```python
from build123d import *

# Parameters (mm, degrees)
SKETCH1_R             = 35
BOSS_EXTRUDE1_DEPTH   = 10
CUT_EXTRUDE1_REACH    = 52.498
SKETCH2_R             = 2.05
F_8_0MM_DOWEL_HOLE1_D = 8
M6_CLEARANCE_HOLE1_D  = 6.4


with BuildPart() as part:
    # Sketch1 → Boss-Extrude1 (new body)
    with BuildSketch(Plane(origin=(0, 0, 0), x_dir=(1, 0, 0), z_dir=(0, 1, 0))):
        with Locations(Location((0, 0, 0), (0, 0, 270))):
            Circle(SKETCH1_R)
    extrude(amount=-BOSS_EXTRUDE1_DEPTH)

    # Sketch2 → Cut-Extrude1 (cut, up to next)
    with BuildSketch(Plane(origin=(0, 0, 0), x_dir=(1, 0, 0), z_dir=(0, 1, 0)), mode=Mode.PRIVATE) as cut_extrude1_sk1:
        with Locations(Location((8.660254038, -5, 0), (0, 0, 270))):
            Circle(SKETCH2_R)
    cut_extrude1_tool1 = extrude(cut_extrude1_sk1.sketch, amount=-CUT_EXTRUDE1_REACH, mode=Mode.PRIVATE) & part.part
    # Sketch2 → Cut-Extrude1 (cut, up to next)
    with BuildSketch(Plane(origin=(0, 0, 0), x_dir=(1, 0, 0), z_dir=(0, 1, 0)), mode=Mode.PRIVATE) as cut_extrude1_sk2:
        with Locations(Location((0, 10, 0), (0, 0, 270))):
            Circle(SKETCH2_R)
    cut_extrude1_tool2 = extrude(cut_extrude1_sk2.sketch, amount=-CUT_EXTRUDE1_REACH, mode=Mode.PRIVATE) & part.part
    # Sketch2 → Cut-Extrude1 (cut, up to next)
    with BuildSketch(Plane(origin=(0, 0, 0), x_dir=(1, 0, 0), z_dir=(0, 1, 0)), mode=Mode.PRIVATE) as cut_extrude1_sk3:
        with Locations(Location((-8.660254038, -5, 0), (0, 0, 270))):
            Circle(SKETCH2_R)
    cut_extrude1_tool3 = extrude(cut_extrude1_sk3.sketch, amount=-CUT_EXTRUDE1_REACH, mode=Mode.PRIVATE) & part.part
    add(cut_extrude1_tool1.solids().sort_by_distance((8.660254, 0, 5))[0], mode=Mode.SUBTRACT)
    add(cut_extrude1_tool2.solids().sort_by_distance((0, 0, -10))[0], mode=Mode.SUBTRACT)
    add(cut_extrude1_tool3.solids().sort_by_distance((-8.660254, 0, 5))[0], mode=Mode.SUBTRACT)

    # Ø8.0mm Dowel Hole1 (through all)
    with Locations(Plane(origin=(0, -10, 0), x_dir=(-1, 0, 0), z_dir=(0, -1, 0))):
        with Locations((-13.75, 23.815698604), (13.75, -23.815698604)):
            Hole(F_8_0MM_DOWEL_HOLE1_D / 2)

    # M6 Clearance Hole1 (through all)
    with Locations(Plane(origin=(0, -10, 0), x_dir=(-1, 0, 0), z_dir=(0, -1, 0))):
        with Locations((-21.650635095, -12.5), (21.650635095, -12.5), (0, 25)):
            Hole(M6_CLEARANCE_HOLE1_D / 2)


solid = part.part
```
Could you check a few things on this model? Use its own coordinates, in mm. Round coordinates to 2 decimals unless told otherwise and drop trailing zeros. Write each loop counter-clockwise with the first axis right and the second up, starting at its lowest first coordinate (ties: lowest second). Pieces come first, ordered by that corner, then holes.
(1) If I drill on probe 1 along X at (y, z) = (-6.75, -24); probe 2 along X at (y, z) = (-4.75, -26); probe 3 along Z at (x, y) = (-21.5, -3.25), over which ranges is the centre line in solid material (lowest first)?
Findings below:
probe 1: x = -25.48 to -3.04, 3.04 to 9.75, 17.75 to 25.48
probe 2: x = -23.43 to -3.04, 3.04 to 10.4, 17.1 to 23.43
probe 3: z = -27.62 to 9.3, 15.7 to 27.62
(2) Suppose I cut it at B-B on z = -25. Write out the boundary of the cut face in (x, y).
Findings below:
outline: (-24.49, -10) - (-3.2, -10) - (-3.2, 0) - (-24.49, 0) - close; (3.2, -10) - (9.93, -10) - (9.93, 0) - (3.2, 0) - close; (17.57, -10) - (24.49, -10) - (24.49, 0) - (17.57, 0) - close
(3) Thinking about a two-plate mould opening in X: for faces 1 (the face through (-16.924, -4.93, 26.25)), 2 (the face through (-21, -5, -28)), 3 (the face through (24.607, -4.93, 13.726)), 4 (the face through (0, 0, 0)), which applies, +X half, -X half, draft (parallel to the pull), parting line (faces both ways), or undercut?
Findings below:
face 1: undercut
face 2: parting line
face 3: undercut
face 4: draft
(4) Suppose I cut it at D-D on z = -10. Write out the boundary of the cut face in (x, y), and give its area (3 significant figures).
Findings below:
outline: (-33.54, -10) - (-2.05, -10) - (-2.05, 0) - (-33.54, 0) - close; (2.05, -10) - (33.54, -10) - (33.54, 0) - (2.05, 0) - close
area: 630 mm2
(5) Suppose I cut it at A-A on x = 0. Write out the boundary of the cut face in (y, z), and give its area (3 significant figures).
Findings below:
outline: (-10, -35) - (0, -35) - (0, -28.2) - (-10, -28.2) - close; (-10, -21.8) - (0, -21.8) - (0, -12.05) - (-10, -12.05) - close; (-10, -7.95) - (0, -7.95) - (0, 35) - (-10, 35) - close
area: 595 mm2
(6) For pin 1 (3 mm diameter, centred on y = -3.5, z = 2, fed in from +X); pin 2 (2 mm diameter, centred on y = -3.5, z = -12, fed in from -X); pin 3 (1.5 mm diameter, centred on y = -7.5, z = 18.5, fed in from +X), each with a flat end and sliding along its axis, tell me the tip position at first contact or that it passes through.
Findings below:
pin 1: stops at x = 35
pin 2: stops at x = -33.23
pin 3: stops at x = 30.17
(7) Suppose I cut it at C-C on x = 16. Write out the boundary of the cut face in (y, z).
Findings below:
outline: (-10, -31.13) - (0, -31.13) - (0, -27.12) - (-10, -27.12) - close; (-10, -20.51) - (0, -20.51) - (0, 31.13) - (-10, 31.13) - close
